Design review of the part shown in the three views and the two pictorial views. Dimensions are in mm from the part's minimum x, y and z. Round coordinates to 2 decimals unless told otherwise and drop trailing zeros. Order: outer loops, then holes, each group sorted by start corner. A loop starts at its lowest first (then second) coordinate and runs counter-clockwise, first axis right, second up.
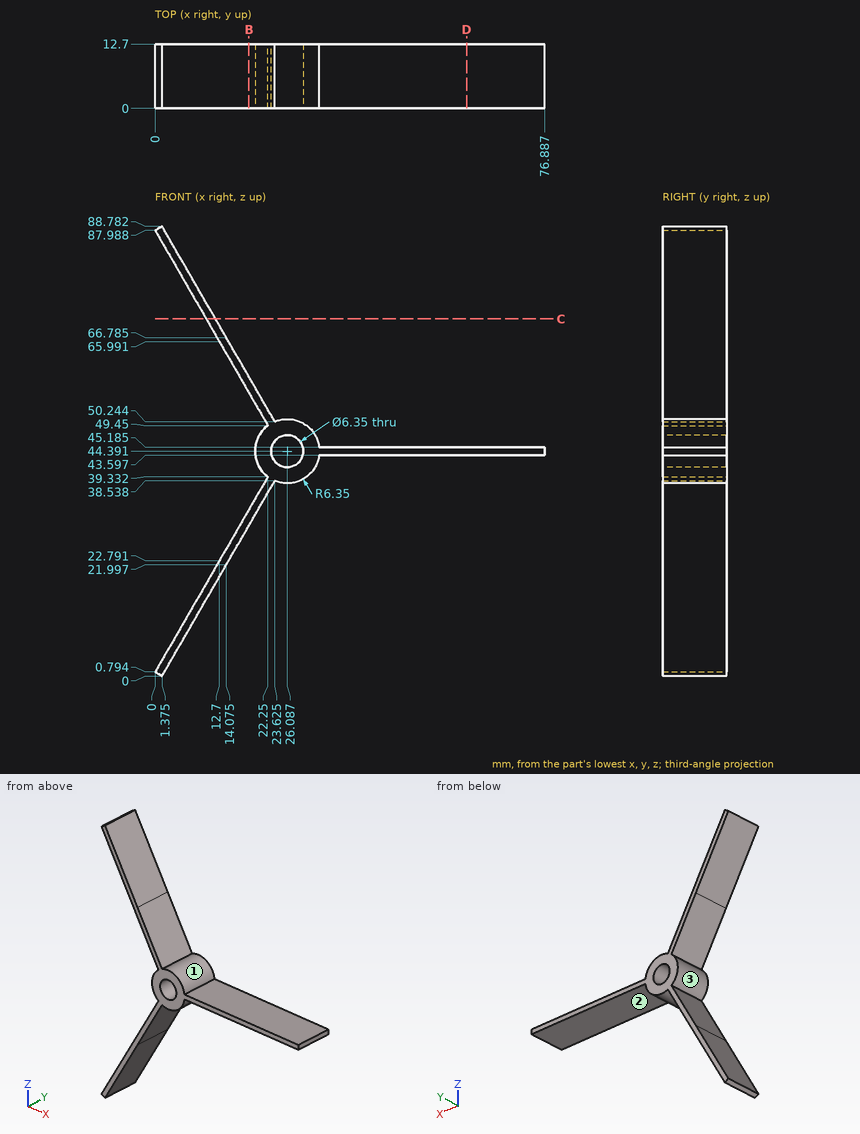
(1) Wall thickness on L1, parallel to Z at x = 20.5, y = 7.25 (1 decimal); L2, parallel to Z at x = 6, y = 8 (1 decimal); L3, parallel to Z at x = 71.5, y = 4.75 (1 decimal): over which ranges is each line inside the solid? List them lowest first.
(2) Add section C-C on z = 70.5. Give the boundary of the cut face in (x, y).
(3) Add section B-B on x = 18.5. Give the boundary of the cut face in (y, z) (1 decimal).
(4) Clearance check with flat-ended pins moving along their axes: P1, Ø4, axis at x = 10, y = 4.5, coming from the +Z side (1 decimal); P2, Ø2, axis at y = 6, z = 63, coming from the -X side; P3, Ø4, axis at x = 54, y = 11, coming from the -Z side. State where each tip first meets the part, or that it passes through.
(5) Draft analysis for pull direction X (two halves, no side actions). For the marked faces 1, 2 and 3, state which applies: pulls with the +X half, pulls with the -X half, needs draft (parallel to the pull), parting line crosses it, or undercut.
(6) Add section D-D on x = 61.5. Give the boundary of the cut face in (y, z) (1 decimal).
Here are the results:
1. L1: z = 33.1 to 36.3, 41.4 to 47.4, 52.5 to 55.7
1. L2: z = 8 to 11.2, 77.6 to 80.8
1. L3: z = 43.6 to 45.2
2. outline: (10.1, 0) - (11.93, 0) - (11.93, 12.7) - (10.1, 12.7) - close
3. outline: (0, 29.7) - (12.7, 29.7) - (12.7, 32.8) - (0, 32.8) - close; (0, 55.9) - (12.7, 55.9) - (12.7, 59.1) - (0, 59.1) - close
4. P1: stops at z = 77.3
4. P2: stops at x = 13.85
4. P3: stops at z = 43.6
5. face 1: undercut
5. face 2: needs draft
5. face 3: pulls with the -X half
6. outline: (0, 43.6) - (12.7, 43.6) - (12.7, 45.2) - (0, 45.2) - close
